Input: dimensioned drawing with shaded views. Units: mm. Origin: part minimum x, y, z. A direction names the side the tool comes from. Round coordinates to 2 decimals unless told otherwise and drop trailing zeros. Write each loop counter-clockwise with the first axis right and the second up, starting at its lowest first coordinate (ties: lowest second). Pieces come first, ordered by that corner, then holes. Notation, with made-up numbers: M 0.25,72.25 L 18.25,72.25 A18 ccw 18.25,97.25 Z; hole C -3.75,87 d6. An arc over 180 degrees is marked long. Answer in a Markdown table with one row per item. Add a question column.
Item 1: Mould query, pull axis Z, two halves, no side actions, for the marked faces 4, 5 and 6. Classes: released by +Z, released by -Z, zero draft, split by the parting line, or undercut.
Item 2: Contact query for a flat-ended pin moving along its axis: pin 1 (1 mm diameter, centred on y = 59, z = 33.5, fed in from -X). Output: stop coordinate, or through.
Item 3: Set-up query: the marked faces 1, 2 and 3. Return all of +Z, -Z, +X, -X, +Y, -Y with unobstructed straight access to the full face (end or side cutting, diameter ignored); none if empty.
Item 4: Cut plane C-C on z = 41. Return loops of the section in (x, y).
Item 5: Cut plane A-A on x = 37. Return loops of the section in (y, z), and give its area (3 significant figures).
Item 6: Cut plane B-B on y = 137.5. Return loops of the section in (x, z), and give its area (3 significant figures).
Item 7: Material intervals for probe 1 along Z at (x, y) = (73, 137); probe 2 along X at (y, z) = (124, 62.5), sorted ascending.
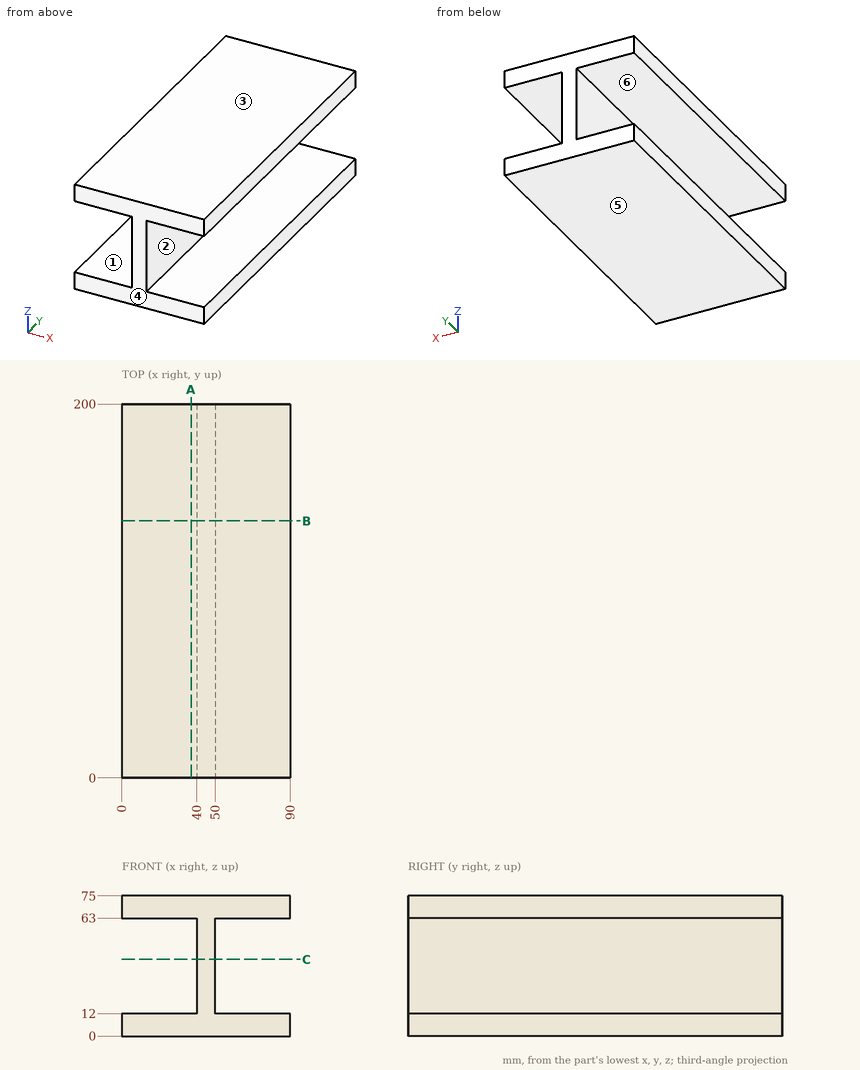
Results below:
| question | item | result |
|---|---|---|
| 1 | face 4 | zero draft |
| 1 | face 5 | released by -Z |
| 1 | face 6 | undercut |
| 2 | pin 1 | x = 40 |
| 3 | face 1 | -X, +Y, -Y |
| 3 | face 2 | +X, +Y, -Y |
| 3 | face 3 | +Z, +X, -X, +Y, -Y |
| 4 | outline | M 40,0 L 50,0 L 50,200 L 40,200 Z |
| 5 | outline | M 0,0 L 200,0 L 200,12 L 0,12 Z; M 0,63 L 200,63 L 200,75 L 0,75 Z |
| 5 | area | 4,800 mm2 |
| 6 | outline | M 0,0 L 90,0 L 90,12 L 50,12 L 50,63 L 90,63 L 90,75 L 0,75 L 0,63 L 40,63 L 40,12 L 0,12 Z |
| 6 | area | 2,670 mm2 |
| 7 | probe 1 | 0 to 12, 63 to 75 |
| 7 | probe 2 | 40 to 50 |
